Geometry: see drawing. Coordinates: mm, zero at the bounding-box minimum. A direction names the side the tool comes from. Round coordinates to 2 decimals unless told otherwise and drop trailing zeros. Loops run counter-clockwise (first coordinate to the right, second up) from the corner with the lowest first, then second, coordinate; pieces in that order, holes last. Notation, with made-up numbers: (29.25, -27.75) - (64.25, -27.75) arc R7 cw to (64.25, -21.75) - close; hole circle Ø4 at (-31.5, -18.5). An arc over 180 degrees is marked (long way). Return JSON: item names as keys, results as strings. Group by question number.
1. First-contact query: pin 1 Ø2.5 at (y, z) = (62.5, 4.5) entering from +X (1 decimal); pin 2 Ø2.5 at (x, z) = (91, 4) entering from +Y. Flat tips, straight axial feed; report the tip coordinate or a pass-through.
2. Set-up query: the marked faces 1, 2, 3 and 4. Return all of +Z, -Z, +X, -X, +Y, -Y with unobstructed straight access to the full face (end or side cutting, diameter ignored); none if empty.
3. Section B-B on x = 44.5. Return loops of the section in (y, z) (1 decimal), and give its area (3 significant figures).
4. Section A-A on y = 28. Return loops of the section in (x, z) (1 decimal), and give its area (3 significant figures).
5. Section D-D on x = 78. Return loops of the section in (y, z), and give its area (3 significant figures).
6. Material intervals for probe 1 along X at (y, z) = (34.5, 7.75) (1 decimal); probe 2 along Y at (x, z) = (28, 4.75) (1 decimal); probe 3 along X at (y, z) = (58, 4.5) (1 decimal), sorted ascending.
7. Section C-C on z = 3. Return loops of the section in (x, y) (1 decimal).
8. Draft query along X for the marked faces 5 and 6. Return one class per face: +X half, -X half, draft (parallel to the pull), parting line (faces both ways), or undercut.
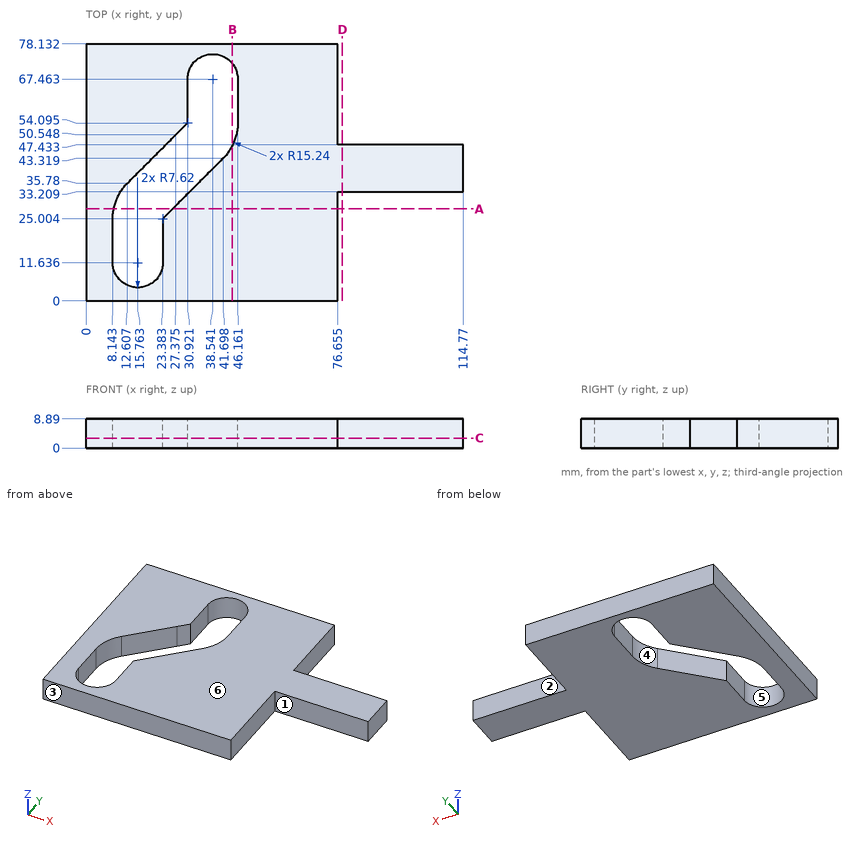
Taken from the geometry:
{
 "1": {"pin 1": "x = 76.7", "pin 2": "y = 47.43"},
 "2": {"face 1": "+Z, -Z, +X, -Y", "face 2": "+Z, -Z, +X, +Y", "face 3": "+Z, -Z, +X, -X, -Y", "face 4": "+Z, -Z"},
 "3": {"outline": "(0, 0) - (47.2, 0) - (47.2, 8.9) - (0, 8.9) - close; (72.2, 0) - (78.1, 0) - (78.1, 8.9) - (72.2, 8.9) - close", "area": "472 mm2"},
 "4": {"outline": "(0, 0) - (8.4, 0) - (8.4, 8.9) - (0, 8.9) - close; (26.4, 0) - (76.7, 0) - (76.7, 8.9) - (26.4, 8.9) - close", "area": "522 mm2"},
 "5": {"outline": "(33.21, 0) - (47.43, 0) - (47.43, 8.89) - (33.21, 8.89) - close", "area": "126 mm2"},
 "6": {"probe 1": "0 to 11.5, 32.9 to 114.8", "probe 2": "0 to 29.6, 51.2 to 78.1", "probe 3": "0 to 30.9, 46.2 to 76.7"},
 "7": {"outline": "(0, 0) - (76.7, 0) - (76.7, 33.2) - (114.8, 33.2) - (114.8, 47.4) - (76.7, 47.4) - (76.7, 78.1) - (0, 78.1) - close; hole (8.1, 11.6) arc R7.6 ccw to (23.4, 11.6) - (23.4, 25) - (41.7, 43.3) arc R15.2 ccw to (46.2, 54.1) - (46.2, 67.5) arc R7.6 ccw to (30.9, 67.5) - (30.9, 54.1) - (27.4, 50.5) - (12.6, 35.8) arc R15.2 ccw to (8.1, 25) - close"},
 "8": {"face 5": "undercut", "face 6": "draft"}
}
